Answer from the drawing. Dimensions are ordinates in mm from the lowest x, y and z of the part. A direction names the side the tool comes from. Give positions to 0.01 mm unless a question says otherwise; leave off trailing zeros. Loops run counter-clockwise (first coordinate to the right, second up) from the corner with the lowest first, then second, coordinate; pieces in that order, holes last.
Item 1: Section B-B, the plane y = 32.5 is taken. Give the vertices of the cut face in (x, z).
Item 2: Section D-D, the plane x = 114.5 is taken. Give the vertices of the cut face in (y, z).
Item 3: Section A-A, the plane x = 77.5 is taken. Give the vertices of the cut face in (y, z).
Item 4: Consider line 1 along Y through (x, z) = (96, 3.25); line 2 along X through (y, z) = (13, 3); line 3 along Z through (x, y) = (26, 44.5). Determine where each line is inside the solid, lowest interval first.
Item 5: A tool of negligible diameter and unlimited length cuts with its end or side. For the marked faces 4, 5, 6 and 7, from which of +Z, -Z, +X, -X, +Y, -Y can it reach the whole face along a straight path? Write none if from no direction.
Item 6: The mould has two halves that part along X. Classify the marked faces 1, 2 and 3: pulls with the +X half, pulls with the -X half, needs draft (parallel to the pull), parting line crosses it, or undercut.
Item 7: Section C-C, the plane z = 13.75 is taken. Give the vertices of the cut face in (x, y).
Item 8: Each of these flat-tipped pins is pushed along its axis until it touches: pin 1 Ø3.5 at (x, z) = (117, 9.5) entering from -Y; pin 2 Ø3.5 at (y, z) = (39.5, 12) entering from -X; pin 3 Ø4.5 at (y, z) = (2.5, 2) entering from +X. Where does it stop, or does it pass through?
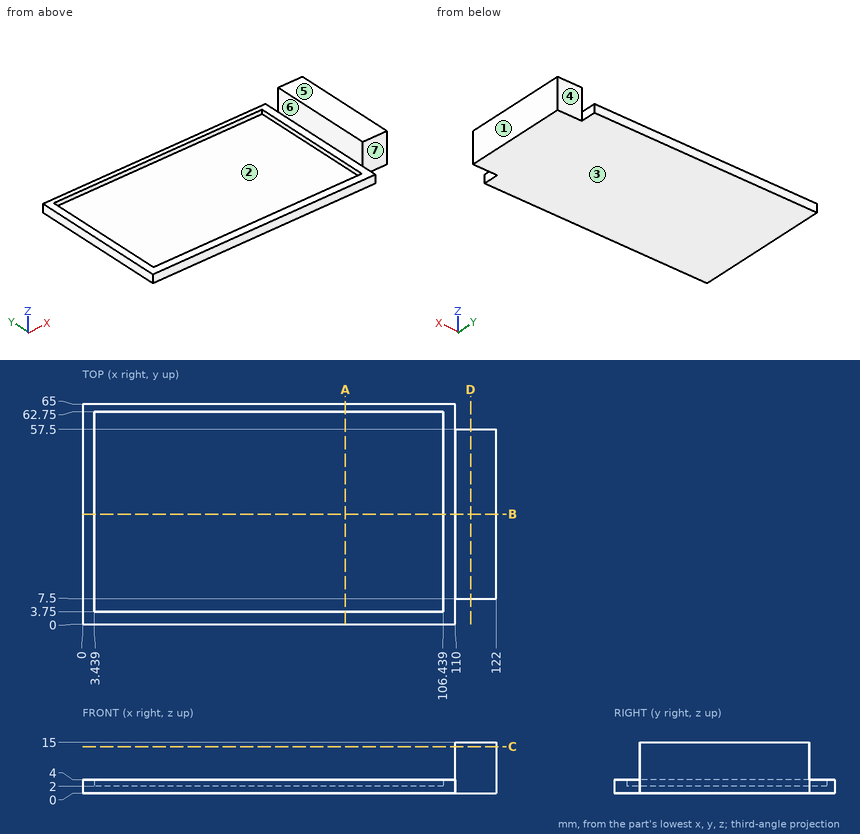
Worked answers:
1. outline: (0, 0) - (122, 0) - (122, 15) - (110, 15) - (110, 4) - (106.44, 4) - (106.44, 2) - (3.44, 2) - (3.44, 4) - (0, 4) - close
2. outline: (7.5, 0) - (57.5, 0) - (57.5, 15) - (7.5, 15) - close
3. outline: (0, 0) - (65, 0) - (65, 4) - (62.75, 4) - (62.75, 2) - (3.75, 2) - (3.75, 4) - (0, 4) - close
4. line 1: y = 0 to 3.75, 62.75 to 65
4. line 2: x = 0 to 3.44, 106.44 to 122
4. line 3: z = 0 to 2
5. face 4: +Z, -Z, +X, +Y
5. face 5: +Z, +X, -X, +Y, -Y
5. face 6: +Z, -X, +Y, -Y
5. face 7: +Z, -Z, +X, -Y
6. face 1: pulls with the +X half
6. face 2: undercut
6. face 3: needs draft
7. outline: (110, 7.5) - (122, 7.5) - (122, 57.5) - (110, 57.5) - close
8. pin 1: stops at y = 7.5
8. pin 2: stops at x = 110
8. pin 3: stops at x = 110
